Geometry check sheet. Reference: the model listing, model coordinates, mm. A direction names the side the tool comes from. Give positions to 0.01 mm unless a question says otherwise; leave off trailing zeros. Write each loop counter-clockwise with the first axis right and the second up, starting at its lowest first coordinate (ties: lowest second). Pieces come first, ordered by that corner, then holes. Notation, with made-up numbers: (48.5, 57.5) -> (65.5, 57.5) arc R19 cw to (65.5, 68.5) -> close; hole circle Ø11 at (68.25, -5.5). An arc over 180 degrees is marked (long way). Write item = value, one per line. Start each with the question number.
1. Thickness scan on line 1 along X through (y, z) = (16.75, 0); line 2 along Y through (x, z) = (-3.75, 1.5); line 3 along Y through (x, z) = (0, 1.5). Record the ranges inside material, lowest first.
2. Cross-section at A-A, the plane z = 0. Record the cut outline in (x, y).
3. Depth check by flat-ended pin: P1, Ø1, axis at y = 10.5, z = 1.5, coming from the +X side; P2, Ø2, axis at y = 16, z = 0.5, coming from the -X side; P3, Ø2, axis at x = -2.5, y = 16.5, coming from the +Z side; P4, Ø2.5, axis at x = 1, z = -1, coming from the +Y side. Enter the tip coordinate at first touch or a pass-through.
4. Set-up check for faces 4 (the cylindrical face through (-2.44, 19.1, -0.54)), 5 (the flat face through (0, 0, 0)): record each of +Z, -Z, +X, -X, +Y, -Y from which the full face is reachable in a straight line by a thin tool's end or side.
5. Cross-section at B-B, the plane y = 21.5. Record the cut outline in (x, z).
6. Cross-section at D-D, the plane z = -3.25. Record the cut outline in (x, y), plus the area to 3 significant figures.
7. Cross-section at C-C, the plane y = 2.5. Record the cut outline in (x, z).
8. Mould release check, pull along Z, two halves, no side actions. Record for faces 1 (the cylindrical face through (0.9, 12.83, 2.86)), 2 (the flat face through (-1, 25, -3)), 3 (the flat face through (0, 12, 0)): pulls with the +Z half, pulls with the -Z half, needs draft (parallel to the pull), parting line crosses it, or undercut.
```python
from build123d import *

# Parameters (mm, degrees)
SKETCH2_R           = 3
BOSS_EXTRUDE1_DEPTH = 26
SKETCH4_R           = 2.5
CUT_EXTRUDE1_DEPTH  = 14
FILLET3_R           = 1
BOSS_EXTRUDE2_START = -1
SKETCH5_R           = 4.25
SKETCH5_R_2         = 3
BOSS_EXTRUDE2_DEPTH = 1


with BuildPart() as part:
    # Sketch2 → Boss-Extrude1 (new body)
    with BuildSketch(Plane(origin=(0, 0, 0), x_dir=(1, 0, 0), z_dir=(0, 1, 0))):
        with Locations(Location((0, 0, 0), (0, 0, 270))):
            Circle(SKETCH2_R)
    extrude(amount=BOSS_EXTRUDE1_DEPTH)

    # Sketch4 → Cut-Extrude1 (cut)
    with BuildSketch(Plane(origin=(0, 26, 0), x_dir=(1, 0, 0), z_dir=(0, 1, 0))):
        with Locations(Location((0, 0, 0), (0, 0, 270))):
            Circle(SKETCH4_R)
    extrude(amount=-CUT_EXTRUDE1_DEPTH, mode=Mode.SUBTRACT)

    # Fillet3
    fillet3_edges = [part.edges().sort_by_distance(p)[0] for p in [
        (0, 0, -3),
    ]]
    fillet(fillet3_edges, radius=FILLET3_R)

    # Sketch5 → Boss-Extrude2 (add)
    with BuildSketch(Plane(origin=(0, 26, 0), x_dir=(1, 0, 0), z_dir=(0, 1, 0)).offset(BOSS_EXTRUDE2_START)):
        with Locations(Location((0, 0, 0), (0, 0, 270))):
            Circle(SKETCH5_R)
        with Locations(Location((0, 0, 0), (0, 0, 270))):
            Circle(SKETCH5_R_2, mode=Mode.SUBTRACT)
    extrude(amount=BOSS_EXTRUDE2_DEPTH)


solid = part.part
```
Answers:
q1.line_1 = -3 to -2.5, 2.5 to 3
q1.line_2 = 25 to 26
q1.line_3 = 0 to 12
q2.outline = (-4.25, 25) -> (-3, 25) -> (-3, 1) arc R1 ccw to (-2, 0) -> (2, 0) arc R1 ccw to (3, 1) -> (3, 25) -> (4.25, 25) -> (4.25, 26) -> (2.5, 26) -> (2.5, 12) -> (-2.5, 12) -> (-2.5, 26) -> (-4.25, 26) -> close
q3.P1 = 2.83
q3.P2 = -3
q3.P3 = 2.6
q3.P4 = 26
q4.face_4 = +Y
q4.face_5 = +Z, -Z, +X, -X, -Y
q5.outline = circle Ø6 at (0, 0); hole circle Ø5 at (0, 0)
q6.outline = (-2.74, 25) -> (2.74, 25) -> (2.74, 26) -> (-2.74, 26) -> close
q6.area = 5.48 mm^2
q7.outline = circle Ø6 at (0, 0)
q8.face_1 = parting line crosses it
q8.face_2 = needs draft
q8.face_3 = undercut
